from build123d import *

# Parameters (mm, degrees)
SKETCH_W                   = 148
SKETCH_H                   = 60
PAD_DEPTH                  = 3
SKETCH002_W                = 138
SKETCH002_H                = 50
SKETCH002_W_2              = 134
SKETCH002_H_2              = 46
PAD001_DEPTH               = 25
SKETCH003_R                = 1.5
POCKET_DEPTH               = 327.272491
PAD002_DEPTH               = 23
SKETCH005_R                = 2.4
POCKET001_DEPTH            = 10
SKETCH003_MIRRORED_2_R     = 1.5
POCKET_MIRRORED_2_DEPTH    = 327.272491
PAD002_MIRRORED_2_DEPTH    = 23
SKETCH005_MIRRORED_2_R     = 2.4
POCKET001_MIRRORED_2_DEPTH = 10


with BuildPart() as part:
    # Sketch → Pad (new body)
    with BuildSketch(Plane.XY):
        Rectangle(SKETCH_W, SKETCH_H)
    extrude(amount=PAD_DEPTH)

    # Sketch002 (on Face5 of Pad) → Pad001 (join)
    with BuildSketch(Plane(origin=(0, 0, 0), x_dir=(1, 0, 0), z_dir=(0, 0, -1))):
        Rectangle(SKETCH002_W, SKETCH002_H)
        Rectangle(SKETCH002_W_2, SKETCH002_H_2, mode=Mode.SUBTRACT)
    extrude(amount=PAD001_DEPTH)

    # Sketch003 (on Face4 of Pad001) → Pocket (cut, through all)
    with BuildSketch(Plane(origin=(0, 0, 0), x_dir=(1, 0, 0), z_dir=(0, 0, -1))):
        with Locations((-71, 27)):
            Circle(SKETCH003_R)
    pocket = extrude(amount=-POCKET_DEPTH, mode=Mode.SUBTRACT)

    # Sketch004 (on Face17 of Pocket) → Pad002 (join)
    with BuildSketch(Plane(origin=(0, 0, 0), x_dir=(1, 0, 0), z_dir=(0, 0, -1))):
        with BuildLine():
            ThreePointArc((-67, 15), (-61.343146, 17.343146), (-59, 23))
            Line((-67, 23), (-59, 23))
            Line((-67, 23), (-67, 15))
        make_face()
    pad002 = extrude(amount=PAD002_DEPTH)

    # Sketch005 (on Face17 of Pad002) → Pocket001 (cut)
    with BuildSketch(Plane(origin=(0, 0, -23), x_dir=(1, 0, 0), z_dir=(0, 0, -1))):
        with Locations((-64, 20)):
            Circle(SKETCH005_R)
    pocket001 = extrude(amount=-POCKET001_DEPTH, mode=Mode.SUBTRACT)

    # Sketch003 Mirrored 2 → Pocket Mirrored 2 (cut, through all)
    with BuildSketch(Plane(origin=(0, 0, 0), x_dir=(-1, 0, 0), z_dir=(0, 0, 1))):
        with Locations((-71, 27)):
            Circle(SKETCH003_MIRRORED_2_R)
    pocket_mirrored_2 = extrude(amount=POCKET_MIRRORED_2_DEPTH, mode=Mode.SUBTRACT)

    # Sketch004 Mirrored 2 → Pad002 Mirrored 2 (add)
    with BuildSketch(Plane(origin=(0, 0, 0), x_dir=(-1, 0, 0), z_dir=(0, 0, 1))):
        with BuildLine():
            ThreePointArc((-67, 15), (-61.343146, 17.343146), (-59, 23))
            Line((-67, 23), (-59, 23))
            Line((-67, 23), (-67, 15))
        make_face()
    pad002_mirrored_2 = extrude(amount=-PAD002_MIRRORED_2_DEPTH)

    # Sketch005 Mirrored 2 → Pocket001 Mirrored 2 (cut)
    with BuildSketch(Plane(origin=(0, 0, -23), x_dir=(-1, 0, 0), z_dir=(0, 0, 1))):
        with Locations((-64, 20)):
            Circle(SKETCH005_MIRRORED_2_R)
    pocket001_mirrored_2 = extrude(amount=POCKET001_MIRRORED_2_DEPTH, mode=Mode.SUBTRACT)

    # Mirrored001: Pocket, Pad002, Pocket001, Pocket Mirrored 2, Pad002 Mirrored 2, Pocket001 Mirrored 2 across Sketch003 H_Axis
    add(pocket.mirror(Plane(origin=(0, 0, 0), x_dir=(0, 0, -1), z_dir=(0, -1, 0))), mode=Mode.SUBTRACT)
    add(pad002.mirror(Plane(origin=(0, 0, 0), x_dir=(0, 0, -1), z_dir=(0, -1, 0))))
    add(pocket001.mirror(Plane(origin=(0, 0, 0), x_dir=(0, 0, -1), z_dir=(0, -1, 0))), mode=Mode.SUBTRACT)
    add(pocket_mirrored_2.mirror(Plane(origin=(0, 0, 0), x_dir=(0, 0, -1), z_dir=(0, -1, 0))), mode=Mode.SUBTRACT)
    add(pad002_mirrored_2.mirror(Plane(origin=(0, 0, 0), x_dir=(0, 0, -1), z_dir=(0, -1, 0))))
    add(pocket001_mirrored_2.mirror(Plane(origin=(0, 0, 0), x_dir=(0, 0, -1), z_dir=(0, -1, 0))), mode=Mode.SUBTRACT)


solid = part.part
The listing builds one solid part. Answer for the finished solid, in the listing's coordinates (mm). A direction names the side the tool comes from. Coordinates: 2 decimals unless noted, no trailing zeros. Order: outer loops, then holes, each group sorted by start corner. A loop starts at its lowest first (then second) coordinate and runs counter-clockwise, first axis right, second up.
Q1. A cutting plane is placed at C-C, the plane x = -71. Write down the section's boundary in (y, z).
Q2. A cutting plane is placed at A-A, the plane y = -27. Write down the section's boundary in (x, z), and give its area (3 significant figures).
Q3. A cutting plane is placed at D-D, the plane y = -4.5. Write down the section's boundary in (x, z).
Q4. A cutting plane is placed at B-B, the plane z = -17.75. Write down the section's boundary in (x, y).
Q5. For a pull along X with two mould halves and no side action, classify faces 3 (the face through (-1, 0, 3)), 4 (the face through (-61.406, -17.281, -11.339)), 5 (the face through (-1, 0, 0)), 6 (the face through (69, 0, -12)) as pulls with the +X half, pulls with the -X half, needs draft (parallel to the pull), parting line crosses it, or undercut.
Q6. Consider line 1 (Y direction, x = 71, z = 0.7); line 2 (Y direction, x = 55, z = -21); line 3 (Y direction, x = -64, z = -17.25). Determine where each line is inside the solid, lowest interval first.
Q7. Which of the six approach directions +Z, -Z, +X, -X, +Y, -Y give full straight-line access (tool end or side, diameter ignored) to faces 1 (the face through (62, 18, -23)), 2 (the face through (70.194, 28.265, 1.479))?
Q8. Given P1, Ø2.5, axis at x = -61, y = -17, coming from the -Z side; P2, Ø1, axis at x = 51, z = -17, coming from the -Y side; P3, Ø4, axis at x = 71, y = 27, coming from the -Z side, each flat-ended and moving along its own axis, determine where each tip first touches the part or whether it passes through.
Answers follow:
1. outline: (-30, 0) - (-28.5, 0) - (-28.5, 3) - (-30, 3) - close; (-25.5, 0) - (25.5, 0) - (25.5, 3) - (-25.5, 3) - close; (28.5, 0) - (30, 0) - (30, 3) - (28.5, 3) - close
2. outline: (-74, 0) - (-72.5, 0) - (-72.5, 3) - (-74, 3) - close; (-69.5, 0) - (69.5, 0) - (69.5, 3) - (-69.5, 3) - close; (72.5, 0) - (74, 0) - (74, 3) - (72.5, 3) - close
2. area: 426 mm2
3. outline: (-74, 0) - (-69, 0) - (-69, -25) - (-67, -25) - (-67, 0) - (67, 0) - (67, -25) - (69, -25) - (69, 0) - (74, 0) - (74, 3) - (-74, 3) - close
4. outline: (-69, -25) - (69, -25) - (69, 25) - (-69, 25) - close; hole (-67, -15) arc R8 cw to (-59, -23) - (59, -23) arc R8 cw to (67, -15) - (67, 15) arc R8 cw to (59, 23) - (-59, 23) arc R8 cw to (-67, 15) - close; hole circle Ø4.8 at (-64, -20); hole circle Ø4.8 at (-64, 20); hole circle Ø4.8 at (64, -20); hole circle Ø4.8 at (64, 20)
5. face 3: needs draft
5. face 4: undercut
5. face 5: undercut
5. face 6: pulls with the +X half
6. line 1: y = -30 to -28.5, -25.5 to 25.5, 28.5 to 30
6. line 2: y = -25 to -23, 23 to 25
6. line 3: y = -25 to -22.4, -17.6 to -15.58, 15.58 to 17.6, 22.4 to 25
7. face 1: -Z
7. face 2: +Z, -Z
8. P1: stops at z = -23
8. P2: stops at y = -25
8. P3: stops at z = 0
